Part model, mm, in its own coordinate system. Face numbers are marked on the shaded views. A direction names the side the tool comes from. Coordinates: 2 decimals unless noted, no trailing zeros. Order: outer loops, then holes, each group sorted by start corner. A loop starts at its lowest first (then second) coordinate and runs counter-clockwise, first axis right, second up.
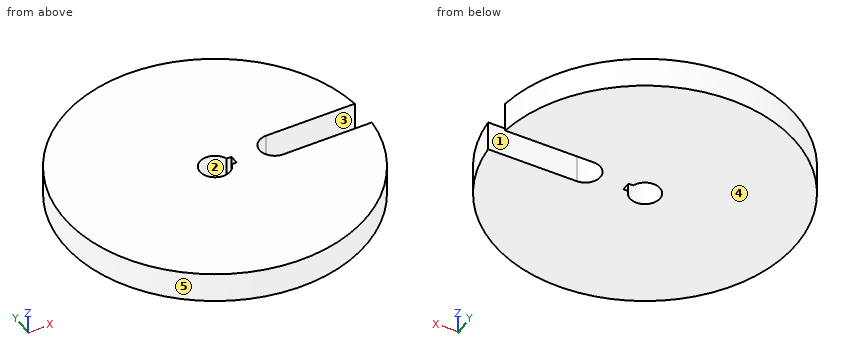
from build123d import *

# Parameters (mm, degrees)
SKETCH_1_R               = 50
EXTRUDE_1_DEPTH          = 10
SKETCH_2_R               = 5
CUT_EXTRUDE_1_DEPTH      = 72.414284285
CUT_EXTRUDE_START        = -1.5
CUT_EXTRUDE_12_OUTLINE_W = 2.4
CUT_EXTRUDE_12_OUTLINE_H = 10
CUT_EXTRUDE_12_DEPTH     = 3
CUT_EXTRUDE_13_DEPTH     = 72.414284285


# Read off the part's stored shape, not the designer's step: 切除-拉伸12
with BuildPart() as part:
    # 草图1 → 凸台-拉伸1 (new body)
    with BuildSketch(Plane.XY):
        Circle(SKETCH_1_R)
    extrude(amount=EXTRUDE_1_DEPTH)

    # 草图2 → 切除-拉伸1 (cut, through all)
    with BuildSketch(Plane.XY.offset(10)):
        Circle(SKETCH_2_R)
    extrude(amount=-CUT_EXTRUDE_1_DEPTH, mode=Mode.SUBTRACT)

    # 切除-拉伸12 outline → 切除-拉伸12 (cut)
    with BuildSketch(Plane(origin=(0, 0, 0), x_dir=(1, 0, 0), z_dir=(0, 1, 0)).offset(CUT_EXTRUDE_START)):
        with Locations((5.2, -5)):
            Rectangle(CUT_EXTRUDE_12_OUTLINE_W, CUT_EXTRUDE_12_OUTLINE_H)
    extrude(amount=CUT_EXTRUDE_12_DEPTH, mode=Mode.SUBTRACT)

    # 草图24 → 切除-拉伸13 (cut, through all)
    with BuildSketch(Plane.XY.offset(10)):
        with BuildLine():
            Line((20, -5), (50, -5))
            ThreePointArc((50, -5), (55, 0), (50, 5))
            Line((50, 5), (20, 5))
            ThreePointArc((20, 5), (15, 0), (20, -5))
        make_face()
    extrude(amount=-CUT_EXTRUDE_13_DEPTH, mode=Mode.SUBTRACT)


solid = part.part
Q1. Mould opens along Y. For the marked faces 3, 4 and 5 say: pulls with the +Y half, pulls with the -Y half, needs draft (parallel to the pull), parting line crosses it, or undercut.
Results list:
face 3: undercut
face 4: needs draft
face 5: parting line crosses it
Q2. Which spindle directions (+Z, -Z, +X, -X, +Y, -Y) get a long thin tool onto all of the face, cutting with end or side? Do the marked faces 1 and 2. Say none if no direction does.
Results list:
face 1: +Z, -Z, +X
face 2: +Z, -Z
Q3. Wall check: line 1 along Y through (x, z) = (0, 7); line 2 along X through (y, z) = (0, 7); line 3 along X through (y, z) = (2, 7.5). Give the ranges that are in metal, low to high.
Results list:
line 1: y = -50 to -5, 5 to 50
line 2: x = -50 to -5, 6.4 to 15
line 3: x = -49.96 to -4.58, 4.58 to 15.42
Q4. Cut at D-D on y = -39.5. Write the cut outline in (x, z), and give its area (3 significant figures).
Results list:
outline: (-30.66, 0) - (30.66, 0) - (30.66, 10) - (-30.66, 10) - close
area: 613 mm2
Q5. Cut at C-C on z = 3. Write the cut outline in (x, y), and give its area (3 significant figures).
Results list:
outline: (20, -5) arc R5 cw to (20, 5) - (49.75, 5) arc R50 ccw (long way) to (49.75, -5) - close; hole (4.77, -1.5) - (6.4, -1.5) - (6.4, 1.5) - (4.77, 1.5) arc R5 ccw (long way) to start
area: 7,430 mm2
Q6. Cut at B-B on x = 0. Write the cut outline in (y, z).
Results list:
outline: (-50, 0) - (-5, 0) - (-5, 10) - (-50, 10) - close; (5, 0) - (50, 0) - (50, 10) - (5, 10) - close
Q7. Cut at A-A on y = 0. Write the cut outline in (x, z).
Results list:
outline: (-50, 0) - (-5, 0) - (-5, 10) - (-50, 10) - close; (6.4, 0) - (15, 0) - (15, 10) - (6.4, 10) - close
Q8. Pin check, flat tips, straight feed: pin 1 Ø1 at (y, z) = (20.5, 4) entering from +X; pin 2 Ø4 at (y, z) = (38.5, 1.5) entering from +X; pin 3 Ø1 at (x, z) = (38, 3) entering from -Y. Stop position of each tip, or through.
Results list:
pin 1: stops at x = 45.83
pin 2: stops at x = 34.17
pin 3: stops at y = -33.07
